The model under review builds one solid part; all positions refer to its coordinate system, in mm. Round coordinates to 2 decimals unless told otherwise and drop trailing zeros. Write each loop counter-clockwise with the first axis right and the second up, starting at its lowest first coordinate (ties: lowest second). Pieces come first, ordered by that corner, then holes. Notation, with made-up numbers: (-29.5, 9) -> (2.5, 9) arc R34 cw to (2.5, 45) -> close; hole circle Ø5 at (77, 69.25). An arc over 180 degrees is marked (long way). Answer as a JSON object with one key per item and string values. Group by question number.
1) We need section B-B, the plane z = -51. Write out the cut boundary in (x, y).
2) We need section C-C, the plane x = -3. Write out the cut boundary in (y, z), then the cut area to 3 significant figures.
3) To check wall thickness, follow probe 1 along X at (y, z) = (0.5, -49); probe 2 along X at (y, z) = (0.3, -12). State the ranges of each line that lie inside material, in increasing order. Write a range as [from, to].
4) We need section A-A, the plane y = 1.3. Write out the cut boundary in (x, z) (3 decimals), then the cut area to 3 significant figures.
5) Insertion check: pin 1 Ø2 at (y, z) = (0.5, -59.5) entering from +X. The pin has a flat end and moves straight along its axis. Give the tip position at first contact, or say it passes through.
from build123d import *

# Parameters (mm, degrees)
SKICA1_R                = 1.75
P_IDAT_VYSUNUT_M1_DEPTH = 3.5


with BuildPart() as part:
    # Skica1 → Přidat vysunutím1 (new body)
    # profile 1 of 2: a face of its own
    with BuildSketch(Plane(origin=(0, 0, 0), x_dir=(1, 0, 0), z_dir=(0, 1, 0))):
        with BuildLine():
            Line((-2, 82), (-3.995243757, 0.195005945))
            ThreePointArc((-3.995243757, 0.195005945), (0, 4), (3.995243757, 0.195005945))
            Line((3.995243757, 0.195005945), (2, 82))
            Line((2, 82), (0, 87.656854249))
            Line((0, 87.656854249), (-2, 82))
        make_face()
    # profile 2 of 2: a face of its own
    with BuildSketch(Plane(origin=(0, 0, 0), x_dir=(1, 0, 0), z_dir=(0, 1, 0))):
        with BuildLine():
            Line((-3.995243757, 0.195005945), (-4, 0))
            ThreePointArc((-4, 0), (0, -4), (4, 0))
            Line((4, 0), (3.995243757, 0.195005945))
            ThreePointArc((3.995243757, 0.195005945), (0, 4), (-3.995243757, 0.195005945))
        make_face()
        with Locations(Location((0, 0, 0), (0, 0, 270))):
            Circle(SKICA1_R, mode=Mode.SUBTRACT)
    extrude(amount=P_IDAT_VYSUNUT_M1_DEPTH)


solid = part.part
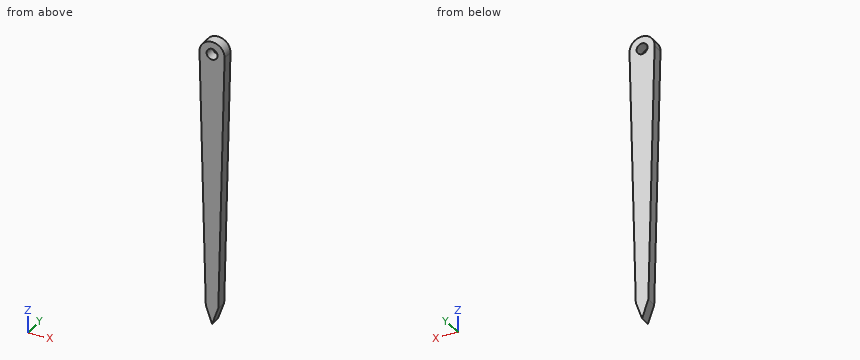
Here are the results:
{
 "1": {"outline": "(-2.76, 0) -> (2.76, 0) -> (2.76, 3.5) -> (-2.76, 3.5) -> close"},
 "2": {"outline": "(0, -41) -> (3.5, -41) -> (3.5, 2.65) -> (0, 2.65) -> close", "area": "153 mm^2"},
 "3": {"probe 1": "x = [-2.8, 2.8]", "probe 2": "x = [-3.71, 3.71]"},
 "4": {"outline": "(-4, 0) -> (-2, -82) -> (0, -87.657) -> (2, -82) -> (4, 0) arc R4 ccw to start; hole circle Ø3.5 at (0, 0)", "area": "519 mm^2"},
 "5": {"pin 1": "stops at x = 2.57"}
}
